Check sheet for the modelled part. Datum: model origin and axes. Units: mm. A direction names the side the tool comes from. Round coordinates to 2 decimals unless told otherwise and drop trailing zeros. Write each loop counter-clockwise with the first axis right and the second up, starting at its lowest first coordinate (ties: lowest second). Pieces come first, ordered by that corner, then holes.
Item 1: Section check A-A, the plane z = 1.5. Record the cut outline in (x, y), plus the area to 3 significant figures.
Item 2: Set-up check for faces 1 (the flat face through (8, 0, 8)), 2 (the flat face through (15, 10, 5)): record each of +Z, -Z, +X, -X, +Y, -Y from which the full face is reachable in a straight line by a thin tool's end or side.
Item 3: Section check B-B, the plane y = 3.75. Record the cut outline in (x, z).
Item 4: Release check for a two-part mould opening along Z. For faces 3 (the flat face through (15, 5, 10)), 4 (the flat face through (5, 30, 10)), 5 (the flat face through (8, 12, 0)) record: pulls with the +Z half, pulls with the -Z half, needs draft (parallel to the pull), parting line crosses it, or undercut.
Item 5: Depth check by flat-ended pin: pin 1 (11 mm diameter, centred on x = 16, z = 6.5, fed in from +Y); pin 2 (1.5 mm diameter, centred on y = 25.5, z = 18, fed in from +X). Enter the tip coordinate at first touch or a pass-through.
Item 6: Material ranges on line 1 along Y through (x, z) = (17, 5), recorded low to high.
Item 7: Section check C-C, the plane x = 11.25. Record the cut outline in (y, z), plus the area to 3 significant figures.
Item 8: Section check D-D, the plane z = 12.75. Record the cut outline in (x, y).
from build123d import *

# Parameters (mm, degrees)
BOX001_W     = 10
BOX001_H     = 10
BOX001_DEPTH = 10
BOX_W        = 10
BOX_H        = 30
BOX_DEPTH    = 20


with BuildPart() as cub001:
    # Box001 → Box001 (new body)
    with BuildSketch(Plane(origin=(10, 0, 0), x_dir=(1, 0, 0), z_dir=(0, 0, 1))):
        with Locations((5, 5)):
            Rectangle(BOX001_W, BOX001_H)
    extrude(amount=BOX001_DEPTH)


with BuildPart() as fusion:
    # Box → Box (new body)
    with BuildSketch(Plane.XY):
        with Locations((5, 15)):
            Rectangle(BOX_W, BOX_H)
    extrude(amount=BOX_DEPTH)

    # Fusion: union Cub001
    add(cub001.part)


solid = fusion.part
Values found:
1. outline: (0, 0) - (20, 0) - (20, 10) - (10, 10) - (10, 30) - (0, 30) - close
1. area: 400 mm2
2. face 1: +Z, -Z, +X, -X, -Y
2. face 2: +Z, -Z, +X, +Y
3. outline: (0, 0) - (20, 0) - (20, 10) - (10, 10) - (10, 20) - (0, 20) - close
4. face 3: pulls with the +Z half
4. face 4: needs draft
4. face 5: pulls with the -Z half
5. pin 1: stops at y = 10
5. pin 2: stops at x = 10
6. line 1: y = 0 to 10
7. outline: (0, 0) - (10, 0) - (10, 10) - (0, 10) - close
7. area: 100 mm2
8. outline: (0, 0) - (10, 0) - (10, 30) - (0, 30) - close
